Geometry check sheet. Reference: the model listing, model coordinates, mm. Round coordinates to 2 decimals unless told otherwise and drop trailing zeros. Order: outer loops, then holes, each group sorted by start corner. A loop starts at its lowest first (then second) coordinate and runs counter-clockwise, first axis right, second up.
(1) Cross-section at C-C on x = 3. Count the separate pieces of the cut face and the enclosed holes in it, and give its area (3 significant figures).
(2) Cross-section at A-A on z = -255. Enter the section's corners in (x, y), and give its area (3 significant figures).
(3) Draft check along Z on faces 1 (the face through (4, 28, 0)), 2 (the face through (4, 27, -300)), 3 (the face through (3.94, 20.31, -267.89)). Enter one of: pulls with the +Z half, pulls with the -Z half, needs draft (parallel to the pull), parting line crosses it, or undercut.
(4) Cross-section at D-D on z = -39. Enter the section's corners in (x, y).
(5) Gauge pin test, flat ends, axial feed: P1, Ø2.5, axis at y = 6.5, z = -270.5, coming from the -X side; P2, Ø5, axis at y = 6.5, z = -29.48, coming from the +X side. Record the tip position at first contact, or that the pin passes through.
(6) Thickness scan on L1, parallel to Z at x = 7.25, y = 21.5; L2, parallel to Z at x = 5.75, y = 6.5; L3, parallel to Y at x = 2.5, z = -270.5. Record the ranges inside material, lowest first.
(7) Cross-section at B-B on y = 25. Enter the section's corners in (x, z), and give its area (3 significant figures).
Autodesk Inventor part; units mm, degrees
ref_plane "YZ Plane" through (0, 0, 0) normal (1, 0, 0) x (0, 1, 0)
ref_plane "XZ Plane" through (0, 0, 0) normal (0, 1, 0) x (-1, 0, 0)
ref_plane "XY Plane" through (0, 0, 0) normal (0, 0, 1) x (1, 0, 0)
sketch "Szkic1" plane through (0, 0, 0) normal (1, 0, 0) x (0, 1, 0)
  line L0 (0, -300) -> (55, -300)
  line L1 (55, 0) -> (0, 0)
  line L2 (55, 0) -> (55, -300)
  circle A0 centre (22, -45) radius 13
  circle A1 centre (22, -255) radius 13
  line L3 (0, 0) -> (0, -300)
  circle A2 centre (37.5154, -29.5) radius 1.5
  circle A3 centre (6.5, -29.4846) radius 1.5
  circle A4 centre (6.4846, -60.5) radius 1.5
  circle A5 centre (37.5, -60.5154) radius 1.5
  circle A6 centre (6.5, -270.5) radius 1.5
  circle A7 centre (37.5, -270.5) radius 1.5
  circle A8 centre (37.5, -239.5) radius 1.5
  circle A9 centre (6.5, -239.5) radius 1.5
  dimension "d0" = 300
  dimension "d1" = 55
  dimension "d2" = 300
  dimension "d5" = 26
  dimension "d8" = 26
  dimension "d9" = 3
  dimension "d12" = 360
  dimension "d14" = 3
  dimension "d17" = 360
extrude "Wyciągnięcie proste1" add sketch "Szkic1" along normal blind 8
properties part number "bok"
Found:
1. separate pieces: 1
1. enclosed holes: 10
1. area: 15,400 mm2
2. outline: (0, 0) - (8, 0) - (8, 9) - (0, 9) - close; (0, 35) - (8, 35) - (8, 55) - (0, 55) - close
2. area: 232 mm2
3. face 1: pulls with the +Z half
3. face 2: pulls with the -Z half
3. face 3: undercut
4. outline: (0, 0) - (8, 0) - (8, 10.47) - (0, 10.47) - close; (0, 33.53) - (8, 33.53) - (8, 55) - (0, 55) - close
5. P1: passes through
5. P2: stops at x = 8
6. L1: z = -300 to -267.99, -242.01 to -57.99, -32.01 to 0
6. L2: z = -300 to -272, -269 to -241, -238 to -62, -59 to -30.98, -27.98 to 0
6. L3: y = 0 to 5, 8 to 36, 39 to 55
7. outline: (0, -300) - (8, -300) - (8, -267.65) - (0, -267.65) - close; (0, -242.35) - (8, -242.35) - (8, -57.65) - (0, -57.65) - close; (0, -32.35) - (8, -32.35) - (8, 0) - (0, 0) - close
7. area: 2,000 mm2
